Design review of the part built by this model. Coordinates are the model's own, in mm. A direction names the side the tool comes from. Round coordinates to 2 decimals unless told otherwise and drop trailing zeros. Loops run counter-clockwise (first coordinate to the right, second up) from the corner with the lowest first, then second, coordinate; pieces in that order, holes last. Notation, with made-up numbers: (2.25, -10) - (37.25, -10) arc R34 ccw to (37.25, 28) - close; hole circle Ø10 at (-25, 14.5). An arc over 180 degrees is marked (long way). Return JSON: item names as keys, results as strings. Group by question number.
from build123d import *

# Parameters (mm, degrees)
SKETCH2_W = 2
SKETCH2_H = 6


with BuildPart() as part:
    # Sweep1: sweep along a path in Sketch1
    with BuildLine(Plane(origin=(0, 0, 0), x_dir=(1, 0, 0), z_dir=(0, 1, 0))) as sweep1_path:
        Line((787.522377583, -234.011074688), (787.522377583, -330.011074688))
        ThreePointArc((787.522377583, -330.011074688), (763.522377583, -354.011074688), (739.522377583, -330.011074688))
        Line((739.522377583, -330.011074688), (739.522377583, -234.011074688))
        ThreePointArc((739.522377583, -234.011074688), (763.522377583, -210.011074688), (787.522377583, -234.011074688))
    # Sketch2 → Sweep1 (sweep)
    with BuildSketch(Plane(origin=(739.522377583, 0, 234.011074688), x_dir=(-1, 0, 0), z_dir=(0, 0, -1))):
        Rectangle(SKETCH2_W, SKETCH2_H)
    sweep(path=sweep1_path.line)


solid = part.part
Q1. Tool access review of faces 5 (the flat face through (740, 3, 277)), 6 (the flat face through (786.522, 0, 283)): name each direction out of +Z, -Z, +X, -X, +Y, -Y from which nothing blocks a thin tool from reaching the whole face with its end or side.
Q2. Add section C-C, the plane y = 0.3. State the section outline as (x, z) points.
Q3. Add section B-B, the plane x = 779. State the section outline as (y, z) points, plus the area to 3 significant figures.
Q4. For line 1 (X direction, y = 0.65, z = 321.5); line 2 (Z direction, x = 764, y = -1.85); line 3 (Z direction, x = 775, y = -2.3), list the stretches that pass through material, from the lowest coordinate up.
Q5. Add section A-A, the plane z = 294. State the section outline as (x, y) points, plus the area to 3 significant figures.
Q6. Draft analysis for pull direction X (two halves, no side actions). For faces 1 (the cylindrical face through (763.017, -0.042, 211.017)), 2 (the flat face through (738.522, 0, 281)), 3 (the flat face through (788.522, 0, 283)), 4 (the flat face through (787, -3, 277)), state which applies: pulls with the +X half, pulls with the -X half, needs draft (parallel to the pull), parting line crosses it, or undercut.
Evaluation:
{
 "1": {"face 5": "+Z, -Z, +X, -X, +Y", "face 6": "+Y, -Y"},
 "2": {"outline": "(738.52, 234.01) arc R25 ccw to (788.52, 234.01) - (788.52, 330.01) arc R25 ccw to (738.52, 330.01) - close; hole (740.52, 234.01) arc R23 ccw to (786.52, 234.01) - (786.52, 330.01) arc R23 ccw to (740.52, 330.01) - close"},
 "3": {"outline": "(-3, 214.38) - (3, 214.38) - (3, 217) - (-3, 217) - close; (-3, 347.02) - (3, 347.02) - (3, 349.64) - (-3, 349.64) - close", "area": "31.4 mm²"},
 "4": {"line 1": "738.52 to 740.52, 786.52 to 788.52", "line 2": "209.02 to 211.02, 353.01 to 355.01", "line 3": "211.8 to 214.08, 349.94 to 352.22"},
 "5": {"outline": "(738.52, -3) - (740.52, -3) - (740.52, 3) - (738.52, 3) - close; (786.52, -3) - (788.52, -3) - (788.52, 3) - (786.52, 3) - close", "area": "24.0 mm²"},
 "6": {"face 1": "undercut", "face 2": "pulls with the -X half", "face 3": "pulls with the +X half", "face 4": "needs draft"}
}
